For this review, take the finished solid that the model builds, in its own axes (mm). Face numbers are marked on the shaded views. A direction names the side the tool comes from. Give positions to 0.01 mm unless a question says otherwise; leave off trailing zeros. Write each loop counter-clockwise with the first axis right and the second up, starting at its lowest first coordinate (ties: lowest second). Pieces come first, ordered by that corner, then holes.
Q1. We need section C-C (y = 40). Write out the cut boundary in (x, z).
Q2. We need section D-D (y = 23). Write out the cut boundary in (x, z).
Q3. We need section A-A (x = 0). Write out the cut boundary in (y, z), then the cut area to 3 significant figures.
Q4. We need section B-B (z = 0). Write out the cut boundary in (x, y), then the cut area to 3 significant figures.
Q5. Machinability: for the marked faces 1 and 2, which of the approach directions +Z, -Z, +X, -X, +Y, -Y give a long, thin tool a straight path to every point of the face, cutting with its end or side? Answer none if there is none.
Q6. Insertion check: P1, Ø1.8, axis at y = 40, z = 0, coming from the +X side; P2, Ø1.7, axis at y = 3, z = 1.5, coming from the +X side; P3, Ø3, axis at y = 47, z = 1.5, coming from the -X side; P4, Ø3, axis at x = -2, y = 48.5, coming from the -Z side. Each pin has a flat end and moves straight along its axis. Give the tip position at first contact, or say it passes through.
Q7. For line 1 (Y direction, x = -0.5, z = 0); line 2 (Z direction, x = 0, y = 40); line 3 (Y direction, x = 0.75, z = 0.75), list the stretches that pass through material, from the lowest coordinate up.
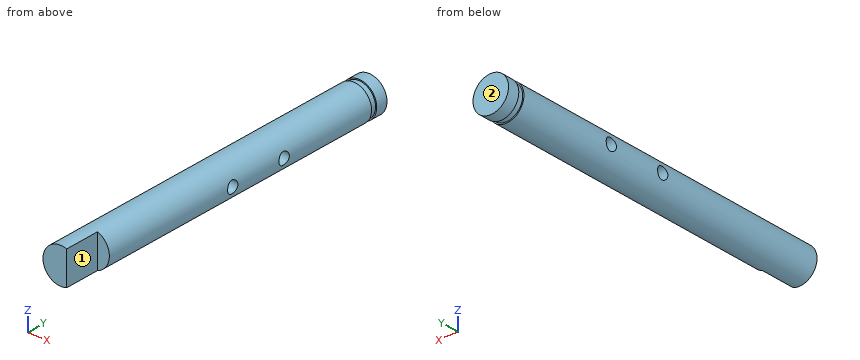
```python
from build123d import *

# Parameters (mm, degrees)
CROQUIS1_R                 = 3
SALIENTE_EXTRUIR1_DEPTH    = 60
CROQUIS2_W                 = 5.531234996
CROQUIS2_H                 = 1
CORTAR_EXTRUIR1_DEPTH      = 61.149812967
CORTAR_EXTRUIR1_DEPTH_BACK = 61.149812967
CROQUIS3_R                 = 1
CORTAR_EXTRUIR2_DEPTH      = 6


with BuildPart() as part:
    # Croquis1 → Saliente-Extruir1 (new body)
    with BuildSketch(Plane(origin=(0, 0, 0), x_dir=(1, 0, 0), z_dir=(0, 1, 0))):
        with Locations(Location((0, 0, 0), (0, 0, 270))):
            Circle(CROQUIS1_R)
    extrude(amount=SALIENTE_EXTRUIR1_DEPTH)

    # Croquis2 → Cortar-Revolución1 (revolve, cut)
    with BuildSketch(Plane.XY, mode=Mode.PRIVATE) as cortar_revoluci_n1_sk:
        with Locations((5.565617498, 57.5)):
            Rectangle(CROQUIS2_W, CROQUIS2_H)
    revolve(cortar_revoluci_n1_sk.sketch.rotate(Axis((0, 60, 0), (0, -1, 0)), 90), axis=Axis((0, 60, 0), (0, -1, 0)), mode=Mode.SUBTRACT)

    # Croquis3 → Cortar-Extruir1 (cut, two sides: drawn at the far end of the back side and taken through both)
    with BuildSketch(Plane(origin=(0, 0, 0), x_dir=(0, 0, -1), z_dir=(1, 0, 0)).offset(-CORTAR_EXTRUIR1_DEPTH_BACK)):
        with Locations((0, 40)):
            Circle(CROQUIS3_R)
        with Locations((0, 30)):
            Circle(CROQUIS3_R)
    extrude(amount=CORTAR_EXTRUIR1_DEPTH + CORTAR_EXTRUIR1_DEPTH_BACK, mode=Mode.SUBTRACT)

    # Croquis4 → Cortar-Extruir2 (cut)
    with BuildSketch(Plane.XZ):
        with BuildLine():
            Line((1, 2.828427125), (1, -2.828427125))
            ThreePointArc((1, -2.828427125), (3, 0), (1, 2.828427125))
        make_face()
    extrude(amount=-CORTAR_EXTRUIR2_DEPTH, mode=Mode.SUBTRACT)


solid = part.part
```
Computed:
1. outline: (-2.83, -1) arc R3 ccw to (2.83, -1) - close; (-2.83, 1) - (2.83, 1) arc R3 ccw to start
2. outline: circle Ø6 at (0, 0)
3. outline: (0, -3) - (57, -3) - (57, -2.8) - (58, -2.8) - (58, -3) - (60, -3) - (60, 3) - (58, 3) - (58, 2.8) - (57, 2.8) - (57, 3) - (0, 3) - close; hole circle Ø2 at (30, 0); hole circle Ø2 at (40, 0)
3. area: 353 mm2
4. outline: (-3, 0) - (1, 0) - (1, 6) - (3, 6) - (3, 29) - (-3, 29) - close; (-3, 31) - (3, 31) - (3, 39) - (-3, 39) - close; (-3, 41) - (3, 41) - (3, 57) - (2.8, 57) - (2.8, 58) - (3, 58) - (3, 60) - (-3, 60) - (-3, 58) - (-2.8, 58) - (-2.8, 57) - (-3, 57) - close
4. area: 324 mm2
5. face 1: +Z, -Z, +X, -Y
5. face 2: +Z, -Z, +X, -X, +Y
6. P1: passes through
6. P2: stops at x = 1
6. P3: stops at x = -3
6. P4: stops at z = -2.96
7. line 1: y = 0 to 29, 31 to 39, 41 to 60
7. line 2: z = -3 to -1, 1 to 3
7. line 3: y = 0 to 29.34, 30.66 to 39.34, 40.66 to 60
